Autodesk Inventor part; units mm, degrees
ref_plane "YZ Plane" through (0, 0, 0) normal (1, 0, 0) x (0, 1, 0)
ref_plane "XZ Plane" through (0, 0, 0) normal (0, 1, 0) x (-1, 0, 0)
ref_plane "XY Plane" through (0, 0, 0) normal (0, 0, 1) x (1, 0, 0)
sketch "Sketch1" plane through (0, 0, 0) normal (0, 0, 1) x (1, 0, 0)
  line L0 (0, 0) -> (32.375, 0)
  line L1 (36.5, 0) -> (36.5, -4.125)
  line L2 (36.5, -22.25) -> (0, -22.25)
  line L3 (0, -22.25) -> (0, -11.125)
  line L4 (0, -11.125) -> (36.5, -11.125) construction
  line L5 (0, -11.125) -> (0, 0)
  circle A0 centre (14.5, -11.125) radius 2
  circle A1 centre (5.25, -2.375) radius 1.5
  arc A2 (36.5, -4.125) -> (32.375, 0) centre (32.375, -4.125) ccw
  line L6 (32.375, 0) -> (36.5, 0)
  line L7 (36.5, -4.125) -> (36.5, -22.25)
  arc A3 (32.375, -22.25) -> (36.5, -18.125) centre (32.375, -18.125) ccw
  circle A4 centre (5.25, -19.875) radius 1.5
  circle A5 centre (24.8, -11.125) radius 2.7
  line L8 (22.8334, -9.275) -> (26.7666, -9.275)
  line L9 (26.7666, -12.975) -> (22.8334, -12.975)
  point P0 (36.5, -18.125)
  dimension "d6" = 4
  dimension "d8" = 3
  dimension "d11" = 5.25
  dimension "d12" = 22.25
  dimension "d13" = 8.75
  dimension "d16" = 14.5
  dimension "d17" = 14
  dimension "d18" = 36.5
  dimension "d19" = 3.7
  dimension "d28" = 5.4
  dimension "d29" = 11.7
extrude "Extrusion1" add sketch "Sketch1" along normal mid plane 18.5 contours L0 A2 L7 A3 L2 L3 L5
extrude "Extrusion2" add sketch "Sketch1" along normal mid plane 22.5 contours A0
extrude "Extrusion3" add sketch "Sketch1" along normal mid plane 20.5 contours A5 L9 L8 | L8 A5 | A5 L9
extrude "Extrusion4" add sketch "Sketch1" along normal mid plane 36.5 contours A5 L9 L8
sketch "Sketch2" plane through (0, -22.25, 9.25) normal (-1, 0, 0) x (0, 0, 1)
  point P0 (-9.25, 22.25)
properties part number "TT motor output"
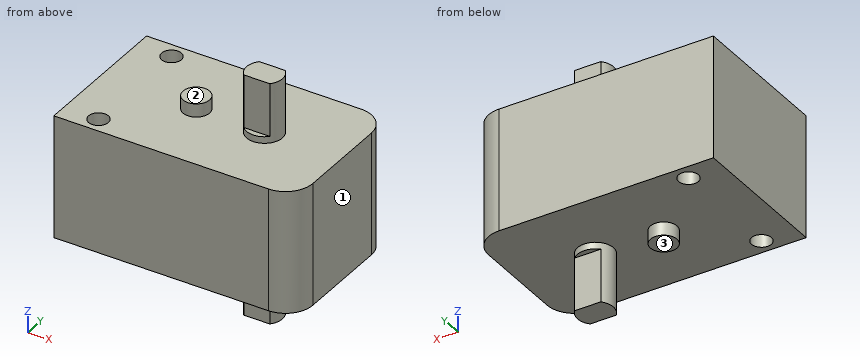
Model file for the job. Use its own axes, mm. Face numbers are marked on the shaded views. A direction names the side the tool comes from. Round coordinates to 2 decimals unless told otherwise and drop trailing zeros. Order: outer loops, then holes, each group sorted by start corner. A loop starts at its lowest first (then second) coordinate and runs counter-clockwise, first axis right, second up.
(1) Band-saw the part on D-D (z = -2). List the corners of the cut face in (x, y) (3 decimals).
(2) Pin check, flat tips, straight feed: pin 1 (0.9 mm diameter, centred on x = 24, y = -13.5, fed in from -Z); pin 2 (0.7 mm diameter, centred on x = 24.5, y = -9, fed in from -Z); pin 3 (3 mm diameter, centred on x = 25.5, z = -12.5, fed in from +Y) (3 decimals); pin 4 (5 mm diameter, centred on x = 30.5, y = -15, fed in from -Z). Stop position of each tip, or through.
(3) Drill centre lines: line 1 (Y direction, x = 5.25, z = 4.5) (3 decimals); line 2 (Z direction, x = 26, y = -6.5); line 3 (X direction, y = -19.25, z = 7). Where is each one in solid material? Low to high.
(4) Band-saw the part on C-C (x = 14.5). List the corners of the cut face in (y, z) (3 decimals).
(5) Band-saw the part on B-B (y = -3). List the corners of the cut face in (x, z).
(6) 3-axis set-ups, long thin cutter, end or side, ignore diameter. For the marked faces 1, 2 and 3: which of +Z, -Z, +X, -X, +Y, -Y reach the whole face in a straight line?
(7) Band-saw the part on A-A (x = 5.25). List the corners of the cut face in (y, z) (3 decimals), then the cut area to 3 significant figures.
Verdict:
1. outline: (0, -22.25) - (32.375, -22.25) arc R4.125 ccw to (36.5, -18.125) - (36.5, -4.125) arc R4.125 ccw to (32.375, 0) - (0, 0) - close; hole circle Ø3 at (5.25, -19.875); hole circle Ø3 at (5.25, -2.375)
2. pin 1: stops at z = -10.25
2. pin 2: stops at z = -18.25
2. pin 3: stops at y = -9.275
2. pin 4: stops at z = -9.25
3. line 1: y = -22.25 to -21.375, -18.375 to -3.875, -0.875 to 0
3. line 2: z = -9.25 to 9.25
3. line 3: x = 0 to 3.89, 6.61 to 36.34
4. outline: (-22.25, -9.25) - (-13.125, -9.25) - (-13.125, -11.25) - (-9.125, -11.25) - (-9.125, -9.25) - (0, -9.25) - (0, 9.25) - (-9.125, 9.25) - (-9.125, 11.25) - (-13.125, 11.25) - (-13.125, 9.25) - (-22.25, 9.25) - close
5. outline: (0, -9.25) - (3.89, -9.25) - (3.89, 9.25) - (0, 9.25) - close; (6.61, -9.25) - (36.34, -9.25) - (36.34, 9.25) - (6.61, 9.25) - close
6. face 1: +Z, -Z, +X, +Y, -Y
6. face 2: +Z, -X, +Y, -Y
6. face 3: -Z, -X, +Y, -Y
7. outline: (-22.25, -9.25) - (-21.375, -9.25) - (-21.375, 9.25) - (-22.25, 9.25) - close; (-18.375, -9.25) - (-3.875, -9.25) - (-3.875, 9.25) - (-18.375, 9.25) - close; (-0.875, -9.25) - (0, -9.25) - (0, 9.25) - (-0.875, 9.25) - close
7. area: 301 mm2
